Geometry check sheet. Reference: the model listing, model coordinates, mm. Face numbers are marked on the shaded views. A direction names the side the tool comes from. Round coordinates to 2 decimals unless told otherwise and drop trailing zeros. Order: outer loops, then holes, each group sorted by start corner. A loop starts at its lowest first (then second) coordinate and runs counter-clockwise, first axis right, second up.
```python
from build123d import *

# Parameters (mm, degrees)
SKETCH1_R               = 17.5
SKETCH1_R_2             = 12.5
EXTRUDE_THIN1_DEPTH     = 12.5
EXTRUDE_THIN1_2_DEPTH   = 12.5
SKETCH2_W               = 186.467509327
SKETCH2_H               = 5
EXTRUDE_THIN2_DEPTH     = 12.5
SKETCH3_W               = 9.044887752
SKETCH3_H               = 4.781773829
CUT_EXTRUDE1_DEPTH      = 13.5
CUT_EXTRUDE1_DEPTH_BACK = 13.5


with BuildPart() as part:
    # Sketch1 → Extrude-Thin1 (new body, symmetric)
    with BuildSketch(Plane.XY):
        with Locations((-66.06, 0)):
            Circle(SKETCH1_R)
        with Locations((-66.06, 0)):
            Circle(SKETCH1_R_2, mode=Mode.SUBTRACT)
    extrude(amount=EXTRUDE_THIN1_DEPTH, both=True)



with BuildPart() as body_2:
    # Sketch1 → Extrude-Thin1 2 (new body, symmetric)
    with BuildSketch(Plane.XY):
        with Locations((66.06, 0)):
            Circle(SKETCH1_R)
        with Locations((66.06, 0)):
            Circle(SKETCH1_R_2, mode=Mode.SUBTRACT)
    extrude(amount=EXTRUDE_THIN1_2_DEPTH, both=True)


with BuildPart() as part_1:
    add(part.part)

    add(body_2.part)  # Extrude-Thin2 merges body 2
    # Sketch2 → Extrude-Thin2 (add, symmetric)
    with BuildSketch(Plane.XY):
        Polygon((-57.1035212, -11.046786298), (0, -60.408556187), (56.960039317, -11.170815772), (53.690229399, -7.388178716), (0, -53.799410338), (-53.833711283, -7.264149241), align=None)
        with Locations((3.112302406, -57.103983263)):
            Rectangle(SKETCH2_W, SKETCH2_H)
    extrude(amount=EXTRUDE_THIN2_DEPTH, both=True)

    # Sketch3 → Cut-Extrude1 (cut, two sides)
    with BuildSketch(Plane.XY) as cut_extrude1_sk:
        with Locations((0.087674805, -61.994870178)):
            Rectangle(SKETCH3_W, SKETCH3_H)
    extrude(amount=CUT_EXTRUDE1_DEPTH, mode=Mode.SUBTRACT)
    extrude(cut_extrude1_sk.sketch, amount=-CUT_EXTRUDE1_DEPTH_BACK, mode=Mode.SUBTRACT)


solid = part_1.part
```
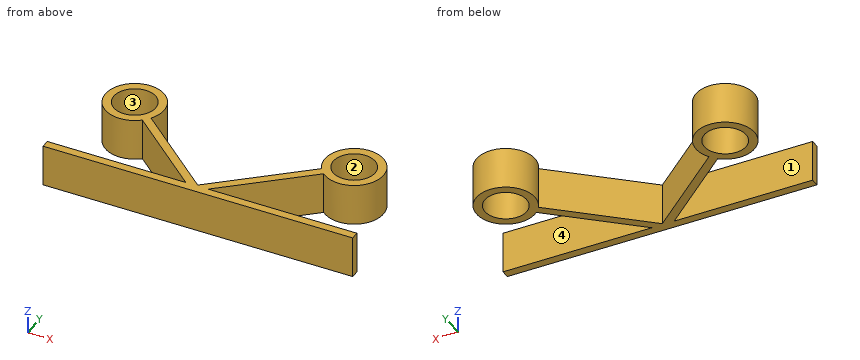
(1) Sectioned sample at A-A, the plane y = 0. Record the cut outline in (x, z).
Returned:
outline: (-83.56, -12.5) - (-78.56, -12.5) - (-78.56, 12.5) - (-83.56, 12.5) - close; (-53.56, -12.5) - (-48.56, -12.5) - (-48.56, 12.5) - (-53.56, 12.5) - close; (48.56, -12.5) - (53.56, -12.5) - (53.56, 12.5) - (48.56, 12.5) - close; (78.56, -12.5) - (83.56, -12.5) - (83.56, 12.5) - (78.56, 12.5) - close
(2) Sectioned sample at B-B, the plane x = -66.06. Record the cut outline in (y, z).
Returned:
outline: (-59.6, -12.5) - (-54.6, -12.5) - (-54.6, 12.5) - (-59.6, 12.5) - close; (-17.5, -12.5) - (-12.5, -12.5) - (-12.5, 12.5) - (-17.5, 12.5) - close; (12.5, -12.5) - (17.5, -12.5) - (17.5, 12.5) - (12.5, 12.5) - close
(3) Material ranges on line 1 (Y direction, x = 66.06, z = -0.75); line 2 (Y direction, x = 69.5, z = 7.5); line 3 (X direction, y = 6.5, z = 10.5), recorded low to high.
Returned:
line 1: y = -59.6 to -54.6, -17.5 to -12.5, 12.5 to 17.5
line 2: y = -59.6 to -54.6, -17.16 to -12.02, 12.02 to 17.16
line 3: x = -82.31 to -76.74, -55.38 to -49.81, 49.81 to 55.38, 76.74 to 82.31
(4) Set-up check for the marked faces 3 and 4: record each of +Z, -Z, +X, -X, +Y, -Y from which the full face is reachable in a straight line by a thin tool's end or side.
Returned:
face 3: +Z, -Z
face 4: +Z, -Z, +X
(5) Sectioned sample at C-C, the plane z = 0. Record the cut outline in (x, y).
Returned:
outline: (-90.12, -59.6) - (96.35, -59.6) - (96.35, -54.6) - (6.71, -54.6) - (54.59, -13.22) arc R17.5 ccw (long way) to (51.32, -9.44) - (0, -53.8) - (-51.32, -9.44) arc R17.5 ccw (long way) to (-54.59, -13.22) - (-6.71, -54.6) - (-90.12, -54.6) - close; hole circle Ø25 at (-66.06, 0); hole circle Ø25 at (66.06, 0)
(6) Depth check by flat-ended pin: P1, Ø2, axis at x = 19, z = -2.5, coming from the +Y side; P2, Ø3, axis at x = 10.5, z = -5, coming from the +Y side; P3, Ø7.5, axis at x = 51.5, z = -1, coming from the +Y side. Enter the tip coordinate at first touch or a pass-through.
Returned:
P1: stops at y = -36.51
P2: stops at y = -43.43
P3: stops at y = 13.76
(7) Draft check along X on the marked faces 1 and 2. Enter one of: released by +X, released by -X, zero draft, split by the parting line, or undercut.
Returned:
face 1: zero draft
face 2: undercut
(8) Sectioned sample at D-D, the plane x = 38. Record the cut outline in (y, z).
Returned:
outline: (-59.6, -12.5) - (-54.6, -12.5) - (-54.6, 12.5) - (-59.6, 12.5) - close; (-27.56, -12.5) - (-20.95, -12.5) - (-20.95, 12.5) - (-27.56, 12.5) - close
